```python
from build123d import *

# Parameters (mm, degrees)
RESSALTO_EXTRUS_O1_DEPTH = 40
ESBO_O2_R                = 1.65
CORTE_EXTRUS_O1_DEPTH    = 40
ESBO_O3_R                = 1.65
CORTE_EXTRUS_O2_DEPTH    = 40


with BuildPart() as part:
    # Esboço1 → Ressalto-extrusão1 (new body)
    with BuildSketch(Plane.XY):
        Polygon((20, 0), (0, 0), (0, 18), (3, 18), (3, 3), (20, 3), align=None)
    extrude(amount=RESSALTO_EXTRUS_O1_DEPTH)

    # Esboço2 → Corte-extrusão1 (cut)
    with BuildSketch(Plane.XZ):
        with Locations((10, 7.5)):
            Circle(ESBO_O2_R)
        with Locations((10, 32.5)):
            Circle(ESBO_O2_R)
    extrude(amount=-CORTE_EXTRUS_O1_DEPTH, mode=Mode.SUBTRACT)

    # Esboço3 → Corte-extrusão2 (cut)
    with BuildSketch(Plane.ZY):
        with Locations((14, 7.5)):
            Circle(ESBO_O3_R)
        with Locations((14, 14.5)):
            Circle(ESBO_O3_R)
    extrude(amount=-CORTE_EXTRUS_O2_DEPTH, mode=Mode.SUBTRACT)


solid = part.part
```
Design review of the part built by this model. Coordinates are the model's own, in mm. A direction names the side the tool comes from. Coordinates: 2 decimals unless noted, no trailing zeros. Order: outer loops, then holes, each group sorted by start corner. A loop starts at its lowest first (then second) coordinate and runs counter-clockwise, first axis right, second up.
1) Take a section at D-D, the plane y = 1.5. Give the boundary of the cut face in (x, z), and give its area (3 significant figures).
2) Mouldability with a two-part tool opening along Y and no side actions: class faces 1 (the cylindrical face through (1.479, 13.868, 15.524)), 2 (the flat face through (1, 18, 20)), 3 (the flat face through (3, 11, 20)) as +Y half, -Y half, draft (parallel to the pull), parting line (faces both ways), or undercut.
3) Take a section at B-B, the plane y = 14.5. Give the boundary of the cut face in (x, z).
4) Wall thickness on line 1 along Y through (x, z) = (1.7, 14); line 2 along Z through (x, y) = (10, 2.2); line 3 along X through (y, z) = (12.75, 19): over which ranges is each line inside the solid? List them lowest first.
5) For faces 4 (the flat face through (11, 3, 20)), 5 (the cylindrical face through (10.89, 1.48, 33.89)), list the 3-axis set-ups (+Z, -Z, +X, -X, +Y, -Y) from which the entire face can be reached by the end or side of a thin tool; tool diameter is ignored.
6) Take a section at C-C, the plane x = 11. Give the boundary of the cut face in (y, z).
7) Clearance check with flat-ended pins moving along their axes: pin 1 (8.5 mm diameter, centred on x = 8, z = 28, fed in from +Y); pin 2 (4.5 mm diameter, centred on y = 14.5, z = 14, fed in from +X); pin 3 (3 mm diameter, centred on x = 10, z = 32.5, fed in from +Y). State where each tip first meets the part, or that it passes through.
8) Take a section at A-A, the plane z = 7.5. Give the boundary of the cut face in (x, y), and give its area (3 significant figures).
Returned:
1. outline: (0, 0) - (20, 0) - (20, 40) - (0, 40) - close; hole circle Ø3.3 at (10, 7.5); hole circle Ø3.3 at (10, 32.5)
1. area: 783 mm2
2. face 1: undercut
2. face 2: +Y half
2. face 3: draft
3. outline: (0, 0) - (3, 0) - (3, 12.35) - (0, 12.35) - close; (0, 15.65) - (3, 15.65) - (3, 40) - (0, 40) - close
4. line 1: y = 0 to 5.85, 9.15 to 12.85, 16.15 to 18
4. line 2: z = 0 to 5.85, 9.15 to 30.85, 34.15 to 40
4. line 3: x = 0 to 3
5. face 4: +Z, -Z, +X, +Y
5. face 5: +Y, -Y
6. outline: (0, 0) - (3, 0) - (3, 6.19) - (0, 6.19) - close; (0, 8.81) - (3, 8.81) - (3, 31.19) - (0, 31.19) - close; (0, 33.81) - (3, 33.81) - (3, 40) - (0, 40) - close
7. pin 1: stops at y = 3
7. pin 2: stops at x = 3
7. pin 3: passes through
8. outline: (0, 0) - (8.35, 0) - (8.35, 3) - (3, 3) - (3, 18) - (0, 18) - close; (11.65, 0) - (20, 0) - (20, 3) - (11.65, 3) - close
8. area: 95.1 mm2
